```python
from build123d import *

# Parameters (mm, degrees)
SKETCH1_R           = 20
BOSS_EXTRUDE1_DEPTH = 800
CHAMFER1_SIZE       = 4
BOSS_EXTRUDE2_START = 280
SKETCH2_R           = 28
BOSS_EXTRUDE2_DEPTH = 40


with BuildPart() as part:
    # Sketch1 → Boss-Extrude1 (new body)
    with BuildSketch(Plane(origin=(0, 0, 0), x_dir=(0, 0, -1), z_dir=(1, 0, 0))):
        Circle(SKETCH1_R)
    extrude(amount=BOSS_EXTRUDE1_DEPTH)

    # Chamfer1
    chamfer1_edges = [part.edges().sort_by_distance(p)[0] for p in [
        (0, 0, 20),
        (800, 0, 20),
    ]]
    chamfer(chamfer1_edges, length=CHAMFER1_SIZE)

    # Sketch2 → Boss-Extrude2 (add)
    with BuildSketch(Plane(origin=(0, 0, 0), x_dir=(0, 0, -1), z_dir=(1, 0, 0)).offset(BOSS_EXTRUDE2_START)):
        Circle(SKETCH2_R)
    extrude(amount=BOSS_EXTRUDE2_DEPTH)


solid = part.part
```
Here's how the part is built. I have some questions about the finished solid (model axes, mm). A direction names the side the tool comes from. Coordinates: 2 decimals unless noted, no trailing zeros. Order: outer loops, then holes, each group sorted by start corner. A loop starts at its lowest first (then second) coordinate and runs counter-clockwise, first axis right, second up. Notation, with made-up numbers: (-32.75, 85.5) - (-6.75, 85.5) arc R28 ccw to (-6.75, 121.5) - close; hole circle Ø11 at (71.25, 15). An arc over 180 degrees is marked (long way). One line per question, with ' | ' between items. Start each with the question number.
1. I'm going to push flat-ended pins straight in: pin 1 Ø2 at (x, y) = (674, -14) entering from +Z; pin 2 Ø4 at (x, y) = (364, 6.5) entering from -Z; pin 3 Ø8 at (y, z) = (9, 19.5) entering from +X; pin 4 Ø8 at (y, z) = (-11.5, -13) entering from -X. Where does each tip first touch, or does it pass through?
2. If we section it at C-C (x = 397): Write out the boundary of the cut face in (y, z).
3. Which directions (+Z, -Z, +X, -X, +Y, -Y) give clear straight access to the entire face, cutting with the end or side of a thin tool? Please do faces 1 (the cylindrical face through (140.068, -19.524, 4.336)), 2 (the cylindrical face through (554.668, -19.524, 4.336)), 3 (the cylindrical face through (299.72, -10.724, -25.865)).
4. If we section it at A-A (z = 0): Write out the boundary of the cut face in (x, y).
5. Please list where these lines run through material, in increasing order: line 1 along X through (y, z) = (25.5, -6.5); line 2 along X through (y, z) = (15, 13); line 3 along Z through (x, y) = (530, 0). Write a range as [from, to].
Model answer:
1) pin 1: stops at z = 15.2 | pin 2: stops at z = -19.49 | pin 3: stops at x = 798.52 | pin 4: stops at x = 0
2) outline: circle Ø40 at (0, 0)
3) face 1: -X | face 2: +X | face 3: +X, -X
4) outline: (0, -16) - (4, -20) - (280, -20) - (280, -28) - (320, -28) - (320, -20) - (796, -20) - (800, -16) - (800, 16) - (796, 20) - (320, 20) - (320, 28) - (280, 28) - (280, 20) - (4, 20) - (0, 16) - close
5) line 1: x = [280, 320] | line 2: x = [3.85, 796.15] | line 3: z = [-20, 20]
